```python
from build123d import *

# Parameters (mm, degrees)
CROQUIS1_W              = 38
CROQUIS1_H              = 19
SALIENTE_EXTRUIR1_DEPTH = 8
CROQUIS2_R              = 5
SALIENTE_EXTRUIR2_DEPTH = 2
CROQUIS3_R              = 3.8
CORTAR_EXTRUIR1_DEPTH   = 24.478713764
CHAFL_N2_SIZE           = 0.7
CROQUIS4_R              = 5.25
CORTAR_EXTRUIR2_DEPTH   = 2.2
CHAFL_N1_SIZE           = 2
CHAFL_N1_SIZE_2         = 3.079729928
CORTAR_EXTRUIR3_START   = -3
CROQUIS6_R              = 8.19764283
CROQUIS6_R_2            = 6.19764283
CORTAR_EXTRUIR3_DEPTH   = 2


with BuildPart() as part:
    # Croquis1 → Saliente-Extruir1 (new body)
    with BuildSketch(Plane(origin=(0, 0, 0), x_dir=(1, 0, 0), z_dir=(0, 1, 0))):
        Rectangle(CROQUIS1_W, CROQUIS1_H)
    extrude(amount=SALIENTE_EXTRUIR1_DEPTH)

    # Croquis2 → Saliente-Extruir2 (add)
    with BuildSketch(Plane(origin=(0, 8, 0), x_dir=(1, 0, 0), z_dir=(0, 1, 0))):
        with Locations(Location((-9.25, 0, 0), (0, 0, 270))):
            Circle(CROQUIS2_R)
        with Locations(Location((9.25, 0, 0), (0, 0, 270))):
            Circle(CROQUIS2_R)
    extrude(amount=SALIENTE_EXTRUIR2_DEPTH)

    # Croquis3 → Cortar-Extruir1 (cut, through all)
    with BuildSketch(Plane(origin=(0, 10, 0), x_dir=(1, 0, 0), z_dir=(0, 1, 0))):
        with Locations(Location((9.25, 0, 0), (0, 0, 270))):
            Circle(CROQUIS3_R)
        with Locations(Location((-9.25, 0, 0), (0, 0, 270))):
            Circle(CROQUIS3_R)
    extrude(amount=-CORTAR_EXTRUIR1_DEPTH, mode=Mode.SUBTRACT)

    # Chaflán2
    chafl_n2_edges = [part.edges().sort_by_distance(p)[0] for p in [
        (-19, 8, 0),
        (0, 8, 9.5),
        (19, 8, 0),
        (0, 0, 9.5),
        (-19, 0, 0),
        (0, 0, -9.5),
        (19, 0, 0),
        (0, 8, -9.5),
        (19, 4, 9.5),
        (-19, 4, 9.5),
        (-19, 4, -9.5),
        (19, 4, -9.5),
    ]]
    chamfer(chafl_n2_edges, length=CHAFL_N2_SIZE)

    # Croquis4 → Cortar-Extruir2 (cut)
    with BuildSketch(Plane.XZ):
        with Locations(Location((9.25, 0, 0), (0, 0, 270))):
            Circle(CROQUIS4_R)
        with Locations(Location((-9.25, 0, 0), (0, 0, 270))):
            Circle(CROQUIS4_R)
    extrude(amount=-CORTAR_EXTRUIR2_DEPTH, mode=Mode.SUBTRACT)

    # Chaflán1
    # the kernel refuses this chamfer: 3.079729928, 2 mm, written as the material it adds along each edge
    with BuildSketch(Plane(origin=(9.25, 8, 0), x_dir=(0, 0, 1), z_dir=(-1, 0, 0))) as chafl_n1_piece_1_section:
        Polygon((5 + CHAFL_N1_SIZE, 0), (5, CHAFL_N1_SIZE_2), (5, 0), align=None)
    chafl_n1_piece_1 = revolve(axis=Axis((9.25, 8, 0), (0, 1, 0)), mode=Mode.PRIVATE)
    chafl_n1_piece_1 = split(chafl_n1_piece_1, bisect_by=Plane(origin=(9.25, 10, -6.344305077), z_dir=(0, -1, 0)), keep=Keep.TOP, mode=Mode.PRIVATE)
    add(chafl_n1_piece_1)
    with BuildSketch(Plane(origin=(-9.25, 8, 0), x_dir=(0, 0, 1), z_dir=(-1, 0, 0))) as chafl_n1_piece_2_section:
        Polygon((5 + CHAFL_N1_SIZE, 0), (5, CHAFL_N1_SIZE_2), (5, 0), align=None)
    chafl_n1_piece_2 = revolve(axis=Axis((-9.25, 8, 0), (0, 1, 0)), mode=Mode.PRIVATE)
    chafl_n1_piece_2 = split(chafl_n1_piece_2, bisect_by=Plane(origin=(-9.25, 10, -6.344305078), z_dir=(0, -1, 0)), keep=Keep.TOP, mode=Mode.PRIVATE)
    add(chafl_n1_piece_2)
    # the kernel refuses this chamfer: 3.079729928, 2 mm, written as the material it takes off along each edge
    with BuildSketch(Plane(origin=(-9.25, 0, 0), x_dir=(0, 0, -1), z_dir=(-1, 0, 0))) as chafl_n1_2_piece_1_section:
        Polygon((5.25 + CHAFL_N1_SIZE, 0), (5.25, -CHAFL_N1_SIZE_2), (5.25, 0), align=None)
    chafl_n1_2_piece_1 = revolve(axis=Axis((-9.25, 0, 0), (0, -1, 0)), mode=Mode.PRIVATE)
    chafl_n1_2_piece_1 = split(chafl_n1_2_piece_1, bisect_by=Plane(origin=(-9.25, 2.2, 6.528205243), z_dir=(0, -1, 0)), keep=Keep.TOP, mode=Mode.PRIVATE)
    add(chafl_n1_2_piece_1, mode=Mode.SUBTRACT)
    with BuildSketch(Plane(origin=(9.25, 0, 0), x_dir=(0, 0, -1), z_dir=(-1, 0, 0))) as chafl_n1_2_piece_2_section:
        Polygon((5.25 + CHAFL_N1_SIZE, 0), (5.25, -CHAFL_N1_SIZE_2), (5.25, 0), align=None)
    chafl_n1_2_piece_2 = revolve(axis=Axis((9.25, 0, 0), (0, -1, 0)), mode=Mode.PRIVATE)
    chafl_n1_2_piece_2 = split(chafl_n1_2_piece_2, bisect_by=Plane(origin=(9.25, 2.2, 6.528205242), z_dir=(0, -1, 0)), keep=Keep.TOP, mode=Mode.PRIVATE)
    add(chafl_n1_2_piece_2, mode=Mode.SUBTRACT)

    # Croquis6 → Cortar-Extruir3 (cut)
    with BuildSketch(Plane(origin=(0, 8, 0), x_dir=(1, 0, 0), z_dir=(0, 1, 0)).offset(CORTAR_EXTRUIR3_START)):
        with Locations((21.250343834, -11.750343834)):
            Circle(CROQUIS6_R)
        with Locations((21.250343834, -11.750343834)):
            Circle(CROQUIS6_R_2, mode=Mode.SUBTRACT)
    extrude(amount=-CORTAR_EXTRUIR3_DEPTH, mode=Mode.SUBTRACT)


solid = part.part
```
Geometry: final body of the model. Coordinates: model frame, mm. A direction names the side the tool comes from. Round coordinates to 2 decimals unless told otherwise and drop trailing zeros. Order: outer loops, then holes, each group sorted by start corner. A loop starts at its lowest first (then second) coordinate and runs counter-clockwise, first axis right, second up. Notation, with made-up numbers: (2.5, 25.25) - (58.5, 25.25) arc R22 cw to (58.5, 31.25) - close; hole circle Ø11 at (64, -18). An arc over 180 degrees is marked (long way). Use CSV: the item, a comma, the result in double quotes. Start each with the question number.
Q1. Section query B-B (x = 9.25). Return loops of the section in (y, z).
Q2. Access query for faces 5 (the face through (-9, 2.2, -4)), 6 (the face through (12.454, 6.155, 2.043)), 7 (the face through (16.893, 4.014, 7.343)). Directions: +Z, -Z, +X, -X, +Y, -Y. A direction counts if a zero-diameter tool reaches every point of the face in a straight line with its end or side. Return the directions, or none.
Q3. Section query A-A (z = 0). State how many separate pieces and enclosed holes the cut face has, and give its area (3 significant figures).
Q4. Material intervals for line 1 along X through (y, z) = (4.5, 0); line 2 along X through (y, z) = (0.5, 1.5); line 3 along Z through (x, y) = (-9, 6.75), sorted ascending. Write a range as from..to.
Q5. Section query D-D (y = 9). Return loops of the section in (x, z), and give its area (3 significant figures).
Q6. First-contact query: pin 1 (3 mm diameter, centred on x = 4, z = -3.5, fed in from -Y); pin 2 (3.5 mm diameter, centred on x = 6.5, z = 1, fed in from -Y); pin 3 (1.7 mm diameter, centred on x = 16, z = 6.5, fed in from +Y). Flat tips, straight axial feed; report the tip coordinate or a pass-through.
Q7. Section query C-C (x = 1.5). Return loops of the section in (y, z), and give its area (3 significant figures).
Q8. Mould query, pull axis X, two halves, no side actions, for faces 1 (the face through (19, 4, 0)), 2 (the face through (-19, 4, 0)), 3 (the face through (-10, 10, -4)), 4 (the face through (-5.48, 6.15, -0.49)). Classes: +X half, -X half, draft (parallel to the pull), parting line (faces both ways), or undercut.
Result set:
1,outline,"(0, -8.8) - (0.7, -9.5) - (7.3, -9.5) - (8, -8.8) - (8, -7) - (10, -5.7) - (10, -3.8) - (2.2, -3.8) - (2.2, -5.82) - (0, -7.25) - close; (0, 7.25) - (2.2, 5.82) - (2.2, 3.8) - (10, 3.8) - (10, 5.7) - (8, 7) - (8, 8.8) - (7.3, 9.5) - (0.7, 9.5) - (0, 8.8) - close"
2,face 5,"-Y"
2,face 6,"+Y, -Y"
2,face 7,"none"
3,separate pieces,"3"
3,enclosed holes,"0"
3,area,"178 mm2"
4,line 1,"x = -19..-13.05, -5.45..5.45, 13.05..19"
4,line 2,"x = -18.8..-16.01, -2.49..2.49, 16.01..18.8"
4,line 3,"z = -9.5..-3.79, 3.79..9.5"
5,outline,"circle Ø12.7 at (-9.25, 0); circle Ø12.7 at (9.25, 0); hole circle Ø7.6 at (-9.25, 0); hole circle Ø7.6 at (9.25, 0)"
5,area,"163 mm2"
6,pin 1,"stops at y = 0"
6,pin 2,"stops at y = 2.2"
6,pin 3,"stops at y = 8"
7,outline,"(0, -8.8) - (0.7, -9.5) - (7.3, -9.5) - (8, -8.8) - (8, 8.8) - (7.3, 9.5) - (0.7, 9.5) - (0, 8.8) - close"
7,area,"151 mm2"
8,face 1,"+X half"
8,face 2,"-X half"
8,face 3,"draft"
8,face 4,"undercut"
